For this review, take the finished solid that the model builds, in its own axes (mm). Face numbers are marked on the shaded views. A direction names the side the tool comes from. Give positions to 0.01 mm unless a question says otherwise; leave off trailing zeros. Write each loop counter-clockwise with the first axis right and the second up, starting at its lowest first coordinate (ties: lowest second). Pieces come first, ordered by that corner, then holes. Notation, with made-up numbers: M 85.5,-7.5 L 111.5,-7.5 A20 ccw 111.5,-1.5 Z; hole C 70.25,-6 d8. An arc over 180 degrees is marked long. One line per item, written item: value. Start each with the question number.
Item 1: Tool access review of the marked faces 4, 5 and 6: name each direction out of +Z, -Z, +X, -X, +Y, -Y from which nothing blocks a thin tool from reaching the whole face with its end or side.
Item 2: Consider section C-C, the plane y = 5.5. Write out the cut boundary in (x, z).
Item 3: Consider section B-B, the plane x = 0. Write out the cut boundary in (y, z).
Item 4: Mouldability with a two-part tool opening along Z and no side actions: class the marked faces 1, 2 and 3 as released by +Z, released by -Z, zero draft, split by the parting line, or undercut.
Item 5: Clearance check with flat-ended pins moving along their axes: pin 1 Ø6 at (x, y) = (5.5, 8) entering from +Z; pin 2 Ø3 at (x, z) = (2.5, -3) entering from +Y; pin 3 Ø5 at (x, y) = (-3, 1.5) entering from -Z. State where each tip first meets the part, or that it passes through.
Item 6: Consider section A-A, the plane z = 0. Write out the cut boundary in (x, y), and give its area (3 significant figures).
Item 7: To check wall thickness, follow probe 1 along X at (y, z) = (4.75, 0); probe 2 along X at (y, z) = (6.75, 1.25). State the ranges of each line that lie inside material, in increasing order.
Item 8: Consider section D-D, the plane y = -2. Write out the cut boundary in (x, z).
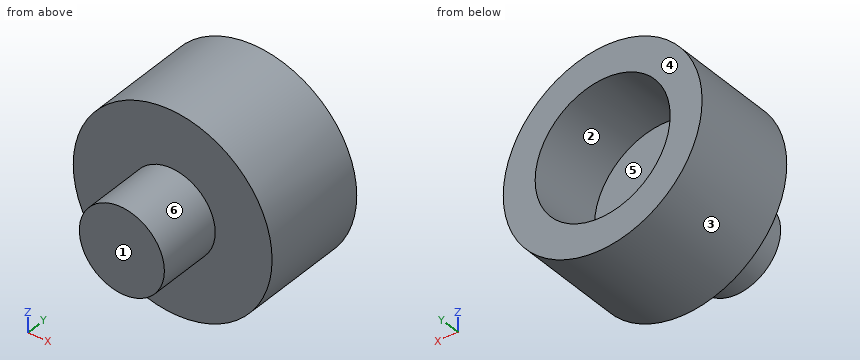
```python
from build123d import *

# Parameters (mm, degrees)
SKETCH1_R           = 9.35
BOSS_EXTRUDE1_DEPTH = 10
SKETCH2_R           = 6.35
CUT_EXTRUDE1_DEPTH  = 7
SKETCH3_R           = 4
BOSS_EXTRUDE2_DEPTH = 6


with BuildPart() as part:
    # Sketch1 → Boss-Extrude1 (new body)
    with BuildSketch(Plane(origin=(0, 0, 0), x_dir=(1, 0, 0), z_dir=(0, 1, 0))):
        Circle(SKETCH1_R)
    extrude(amount=BOSS_EXTRUDE1_DEPTH)

    # Sketch2 → Cut-Extrude1 (cut)
    with BuildSketch(Plane(origin=(0, 10, 0), x_dir=(1, 0, 0), z_dir=(0, 1, 0))):
        Circle(SKETCH2_R)
    extrude(amount=-CUT_EXTRUDE1_DEPTH, mode=Mode.SUBTRACT)

    # Sketch3 → Boss-Extrude2 (add)
    with BuildSketch(Plane.XZ):
        Circle(SKETCH3_R)
    extrude(amount=BOSS_EXTRUDE2_DEPTH)


solid = part.part
```
Model answer:
1. face 4: +Z, -Z, +X, -X, +Y
1. face 5: +Y
1. face 6: -Y
2. outline: C 0,0 d18.7; hole C 0,0 d12.7
3. outline: M -6,-4 L 0,-4 L 0,-9.35 L 10,-9.35 L 10,-6.35 L 3,-6.35 L 3,6.35 L 10,6.35 L 10,9.35 L 0,9.35 L 0,4 L -6,4 Z
4. face 1: zero draft
4. face 2: undercut
4. face 3: split by the parting line
5. pin 1: stops at z = 9.01
5. pin 2: stops at y = 3
5. pin 3: stops at z = -9.34
6. outline: M -9.35,0 L -4,0 L -4,-6 L 4,-6 L 4,0 L 9.35,0 L 9.35,10 L 6.35,10 L 6.35,3 L -6.35,3 L -6.35,10 L -9.35,10 Z
6. area: 146 mm2
7. probe 1: x = -9.35 to -6.35, 6.35 to 9.35
7. probe 2: x = -9.27 to -6.23, 6.23 to 9.27
8. outline: C 0,0 d8
